```python
from build123d import *

# Parameters (mm, degrees)
BASE_FLANGE1_DEPTH       = 480
CUT_EXTRUDE1_START       = -3
SKETCH6_W                = 170
SKETCH6_H                = 41
CUT_EXTRUDE1_DEPTH       = 902.017817195
M5_CLEARANCE_HOLE1_D     = 5.8
FILLET1_R                = 15
M8_CLEARANCE_HOLE1_D     = 10
M8_CLEARANCE_HOLE2_D     = 10
M8_CLEARANCE_HOLE2_DEPTH = 8.995696905
M8_CLEARANCE_HOLE2_TIP   = 3.004303095
M8_CLEARANCE_HOLE3_D     = 10
M8_CLEARANCE_HOLE3_DEPTH = 8.995696905
M8_CLEARANCE_HOLE3_TIP   = 3.004303095


# Sheet-metal steps are written as plain solids
with BuildPart() as part:
    # Sketch1 → Base-Flange1 (new, symmetric)
    with BuildSketch(Plane(origin=(0, 0, 0), x_dir=(1, 0, 0), z_dir=(0, 1, 0))):
        with BuildLine():
            Line((-370.5, 40), (-370.5, 1.5))
            ThreePointArc((-370.5, 1.5), (-370.060660172, 0.439339828), (-369, 0))
            Line((-369, 0), (369, 0))
            ThreePointArc((369, 0), (370.060660172, 0.439339828), (370.5, 1.5))
            Line((370.5, 1.5), (370.5, 150))
            Line((370.5, 150), (372, 150))
            Line((372, 150), (372, 1.5))
            ThreePointArc((372, 1.5), (371.121320344, -0.621320344), (369, -1.5))
            Line((369, -1.5), (-369, -1.5))
            ThreePointArc((-369, -1.5), (-371.121320344, -0.621320344), (-372, 1.5))
            Line((-372, 1.5), (-372, 40))
            Line((-372, 40), (-370.5, 40))
        make_face()
    extrude(amount=BASE_FLANGE1_DEPTH, both=True)

    # Sketch6 → Cut-Extrude1 (cut)
    with BuildSketch(Plane(origin=(372, 0, 0), x_dir=(0, 0, -1), z_dir=(1, 0, 0)).offset(CUT_EXTRUDE1_START)):
        with Locations((73.5, 459.5)):
            Rectangle(SKETCH6_W, SKETCH6_H)
    cut_extrude1 = extrude(amount=CUT_EXTRUDE1_DEPTH, mode=Mode.SUBTRACT)

    # Mirror1: Cut-Extrude1 across plane
    add(cut_extrude1.mirror(Plane.ZX), mode=Mode.SUBTRACT)

    # M5 Clearance Hole1 (through all)
    with Locations(Plane(origin=(372, 0, 0), x_dir=(0, 0, -1), z_dir=(1, 0, 0))):
        with Locations((75.75, 379), (75.75, 189.5), (75.75, 0), (75.75, -189.5), (75.75, -379)):
            Hole(M5_CLEARANCE_HOLE1_D / 2)

    # Fillet1
    fillet1_edges = [part.edges().sort_by_distance(p)[0] for p in [
        (-371.25, -480, -40),
        (369, -480, 0.75),
        (369, 480, 0.75),
        (371.25, 439, -150),
        (371.25, -439, -150),
        (-371.25, 480, -40),
    ]]
    fillet(fillet1_edges, radius=FILLET1_R)

    # M8 Clearance Hole1 (through all)
    with Locations(Plane.XY.offset(1.5)):
        with Locations((349, 460), (116.333333333, 460), (-116.333333333, 460), (-349, 460)):
            m8_clearance_hole1 = Hole(M8_CLEARANCE_HOLE1_D / 2)

    # Mirror2: M8 Clearance Hole1 across plane
    add(m8_clearance_hole1.mirror(Plane.ZX), mode=Mode.SUBTRACT)

    # M8 Clearance Hole2
    with Locations(Plane.ZY.offset(372)):
        with Locations((-20, 410), (-20, 136.666666667), (-20, -136.666666667), (-20, -410)):
            Hole(M8_CLEARANCE_HOLE2_D / 2, depth=M8_CLEARANCE_HOLE2_DEPTH)
            with Locations((0, 0, -(M8_CLEARANCE_HOLE2_DEPTH + M8_CLEARANCE_HOLE2_TIP / 2))):  # 118° drill point
                Cone(0, M8_CLEARANCE_HOLE2_D / 2, M8_CLEARANCE_HOLE2_TIP, mode=Mode.SUBTRACT)

    # M8 Clearance Hole3
    with Locations(Plane(origin=(372, 0, 0), x_dir=(0, 0, -1), z_dir=(1, 0, 0))):
        with Locations((20, 369), (20, 0), (20, -369)):
            Hole(M8_CLEARANCE_HOLE3_D / 2, depth=M8_CLEARANCE_HOLE3_DEPTH)
            with Locations((0, 0, -(M8_CLEARANCE_HOLE3_DEPTH + M8_CLEARANCE_HOLE3_TIP / 2))):  # 118° drill point
                Cone(0, M8_CLEARANCE_HOLE3_D / 2, M8_CLEARANCE_HOLE3_TIP, mode=Mode.SUBTRACT)


solid = part.part
```
Geometry: final body of the model. Coordinates: model frame, mm. A direction names the side the tool comes from. Round coordinates to 2 decimals unless told otherwise and drop trailing zeros. Order: outer loops, then holes, each group sorted by start corner. A loop starts at its lowest first (then second) coordinate and runs counter-clockwise, first axis right, second up. Notation, with made-up numbers: (53, 58) -> (85, 58) arc R11 ccw to (85, 63) -> close; hole circle Ø2 at (25.5, -40). An arc over 180 degrees is marked (long way). Use one line per item in the form item = value. Start each with the question number.
1. Draft query along X for faces 3 (the face through (5, 7, 1.5)), 4 (the face through (372, 6, -77)), 5 (the face through (-5, 7, 0)). Return one class per face: pulls with the +X half, pulls with the -X half, needs draft (parallel to the pull), parting line crosses it, or undercut.
2. Reachability of faces 1 (the face through (-370.5, 7, -21)), 2 (the face through (-7, 480, 1)) from +Z, -Z, +X, -X, +Y, -Y: full face, straight path, thin tool, end or side. Return the list, or none.
3. Cut plane A-A (x = 272). Return the cut outline in (y, z), then the cut area to 3 significant figures.
4. Line query: probe 1 along X at (y, z) = (460, 1.2); probe 2 along Y at (x, z) = (371.25, -20); probe 3 along X at (y, z) = (-55.5, -11.5). Output: solid intervals per line, ascending.
5. Pin query (flat end, axial travel): pin 1 Ø2 at (x, y) = (16.5, 146.5) entering from -Z; pin 2 Ø9 at (y, z) = (-410, -20) entering from -X; pin 3 Ø6 at (x, y) = (-349, -460) entering from -Z; pin 4 Ø1.5 at (x, z) = (371, -99) entering from -Y. Return the tip coordinate at first contact, or that it passes through.
6. Cut plane B-B (z = -53.5). Return the cut outline in (x, y).
Solution:
q1.face_3 = needs draft
q1.face_4 = pulls with the +X half
q1.face_5 = undercut
q2.face_1 = -Z, +Y, -Y
q2.face_2 = +Z, -Z, +X, -X, +Y
q3.outline = (-480, 0) -> (480, 0) -> (480, 1.5) -> (-480, 1.5) -> close
q3.area = 1,440 mm^2
q4.probe_1 = -370.31 to -354, -344 to -121.33, -111.33 to 111.33, 121.33 to 344, 354 to 369
q4.probe_2 = -439 to -374, -364 to -5, 5 to 364, 374 to 439
q4.probe_3 = -372 to -370.5, 370.5 to 372
q5.pin_1 = 0
q5.pin_2 = 370.5
q5.pin_3 = through
q5.pin_4 = -439
q6.outline = (370.5, -439) -> (372, -439) -> (372, 439) -> (370.5, 439) -> close
